Geometry check sheet. Reference: the model listing, model coordinates, mm. A direction names the side the tool comes from. Coordinates: 2 decimals unless noted, no trailing zeros. Order: outer loops, then holes, each group sorted by start corner. A loop starts at its lowest first (then second) coordinate and runs counter-clockwise, first axis right, second up. Notation, with made-up numbers: (0.5, 44) -> (51.5, 44) arc R23 ccw to (51.5, 77) -> close; hole circle Ø7 at (36, 25). An arc over 180 degrees is marked (long way). Answer as CSV lines item,"result". Start each with the question number.
from build123d import *

# Parameters (mm, degrees)
SKETCH1_R           = 12.2
BOSS_EXTRUDE1_DEPTH = 45
SKETCH2_R           = 6
BOSS_EXTRUDE2_DEPTH = 1
SKETCH3_R           = 1.5
BOSS_EXTRUDE3_DEPTH = 8
FILLET1_R           = 3
FILLET2_R           = 1
FILLET3_R           = 0.3
FILLET4_R           = 0.3


with BuildPart() as part:
    # Sketch1 → Boss-Extrude1 (new body)
    with BuildSketch(Plane.XY):
        with Locations(Location((0, 0, 0), (0, 0, 180))):
            Circle(SKETCH1_R)
    extrude(amount=BOSS_EXTRUDE1_DEPTH)

    # Sketch2 → Boss-Extrude2 (add)
    with BuildSketch(Plane.XY.offset(45)):
        Circle(SKETCH2_R)
    extrude(amount=BOSS_EXTRUDE2_DEPTH)

    # Sketch3 → Boss-Extrude3 (add)
    with BuildSketch(Plane.XY.offset(45)):
        Circle(SKETCH3_R)
    extrude(amount=BOSS_EXTRUDE3_DEPTH)

    # Fillet1
    fillet1_edges = [part.edges().sort_by_distance(p)[0] for p in [
        (12.2, 0, 45),
    ]]
    fillet(fillet1_edges, radius=FILLET1_R)

    # Fillet2
    fillet2_edges = [part.edges().sort_by_distance(p)[0] for p in [
        (12.2, 0, 0),
    ]]
    fillet(fillet2_edges, radius=FILLET2_R)

    # Fillet3
    fillet3_edges = [part.edges().sort_by_distance(p)[0] for p in [
        (-6, 0, 45),
        (-6, 0, 46),
    ]]
    fillet(fillet3_edges, radius=FILLET3_R)

    # Fillet4
    fillet4_edges = [part.edges().sort_by_distance(p)[0] for p in [
        (-1.5, 0, 53),
    ]]
    fillet(fillet4_edges, radius=FILLET4_R)


solid = part.part
Q1. Sectioned sample at D-D, the plane z = 34. Record the cut outline in (x, y).
Q2. Sectioned sample at C-C, the plane z = 48. Record the cut outline in (x, y), then the cut area to 3 significant figures.
Q3. Thickness scan on L1, parallel to Z at x = 4.5, y = -1; L2, parallel to X at y = -0.25, z = 15.5; L3, parallel to Z at x = -6, y = -3.5. Record the ranges inside material, lowest first.
Q4. Access from +Z, -Z, +X, -X, +Y, -Y to the whole of each face (thin tool, end or side, straight path). Record for faces 1 (the cylindrical face through (12.19, -0.54, 21.21)), 2 (the flat face through (1.2, -1.2, 46)).
Q5. Go/stop test with flat-tipped pins: pin 1 Ø1 at (x, z) = (5.5, 38) entering from +Y; pin 2 Ø5 at (x, z) = (-5, 8.5) entering from +Y; pin 3 Ø3 at (y, z) = (-9.5, 39) entering from +X. Record where each tip stops, or that it passes through.
Q6. Sectioned sample at A-A, the plane x = 0. Record the cut outline in (y, z), then the cut area to 3 significant figures.
Geometry results:
1,outline,"circle Ø24.4 at (0, 0)"
2,outline,"circle Ø3 at (0, 0)"
2,area,"7.07 mm^2"
3,L1,"z = 0 to 46"
3,L2,"x = -12.2 to 12.2"
3,L3,"z = 0 to 45"
4,face 1,"+Z, -Z"
4,face 2,"+Z"
5,pin 1,"stops at y = 11.13"
5,pin 2,"stops at y = 11.94"
5,pin 3,"stops at x = 9.21"
6,outline,"(-12.2, 1) arc R1 ccw to (-11.2, 0) -> (11.2, 0) arc R1 ccw to (12.2, 1) -> (12.2, 42) arc R3 ccw to (9.2, 45) -> (6.3, 45) arc R0.3 cw to (6, 45.3) -> (6, 45.7) arc R0.3 ccw to (5.7, 46) -> (1.5, 46) -> (1.5, 52.7) arc R0.3 ccw to (1.2, 53) -> (-1.2, 53) arc R0.3 ccw to (-1.5, 52.7) -> (-1.5, 46) -> (-5.7, 46) arc R0.3 ccw to (-6, 45.7) -> (-6, 45.3) arc R0.3 cw to (-6.3, 45) -> (-9.2, 45) arc R3 ccw to (-12.2, 42) -> close"
6,area,"1,130 mm^2"
